The listing builds one solid part. Answer for the finished solid, in the listing's coordinates (mm). Give positions to 0.01 mm unless a question says otherwise; leave off trailing zeros. Order: outer loops, then holes, each group sorted by start corner. A loop starts at its lowest first (then second) coordinate and runs counter-clockwise, first axis right, second up. Notation, with made-up numbers: (27.5, -15.5) -> (55.5, -15.5) arc R17 ccw to (55.5, -3.5) -> close; hole circle Ø10 at (13.25, -13.5). An arc over 180 degrees is marked (long way). Write item = value, one per line. Start each with the question number.
Autodesk Inventor part; units mm, degrees
ref_plane "YZ Plane" through (0, 0, 0) normal (1, 0, 0) x (0, 1, 0)
ref_plane "XZ Plane" through (0, 0, 0) normal (0, 1, 0) x (-1, 0, 0)
ref_plane "XY Plane" through (0, 0, 0) normal (0, 0, 1) x (1, 0, 0)
sketch "スケッチ1" plane through (0, 0, 0) normal (1, 0, 0) x (0, 1, 0)
  circle A0 centre (0, 0) radius 15
  dimension "d0" = 30
extrude "押し出し1" add sketch "スケッチ1" along normal blind 10
sketch "スケッチ2" plane through (10, 0, 0) normal (1, 0, 0) x (0, 0, -1)
  circle A0 centre (0, 0) radius 16
  dimension "d3" = 32
extrude "押し出し2" add sketch "スケッチ2" along normal blind 1
sketch "スケッチ3" plane through (0, 0, 0) normal (-1, 0, 0) x (0, 0, 1)
  circle A0 centre (0, 0) radius 16
  dimension "d6" = 32
extrude "押し出し3" add sketch "スケッチ3" along normal blind 1
sketch "スケッチ4" plane through (-1, 0, 0) normal (-1, 0, 0) x (0, 0, 1)
  circle A0 centre (0, 0) radius 6
  dimension "d9" = 12
extrude "押し出し4" cut sketch "スケッチ4" against normal blind 12
properties part number "type2" material "アセタール樹脂、白"
Item 1: Consider L1, parallel to X at y = -14, z = -5.5; L2, parallel to Y at x = 1.25, z = 4; L3, parallel to Z at x = 8.25, y = -0.5. Determine where each line is inside the solid, lowest interval first. Write a range as from..to.
Item 2: A cutting plane is placed at D-D, the plane y = -12. Write down the section's boundary in (x, z).
Item 3: Flat-ended cylindrical pins translate along their axes: pin 1 (2 mm diameter, centred on x = 6, y = -7.5, fed in from -Z); pin 2 (3 mm diameter, centred on x = 3.5, y = 3, fed in from +Z); pin 3 (4 mm diameter, centred on x = 7, z = 2, fed in from +Y). Find the tip coordinate at first contact, or state that the pin passes through.
Item 4: A cutting plane is placed at A-A, the plane z = 0. Write down the section's boundary in (x, y).
Item 5: A cutting plane is placed at C-C, the plane x = 6. Write down the section's boundary in (y, z).
Item 6: The mould has two halves that part along Y. Classify faces 1 (the flat face through (-1, 0, 7)), 2 (the cylindrical face through (4.93, -14.985, -0.66)), 3 (the cylindrical face through (5, 0, -6)): +Y half, -Y half, draft (parallel to the pull), parting line (faces both ways), or undercut.
Check values:
q1.L1 = -1..0, 10..11
q1.L2 = -14.46..-4.47, 4.47..14.46
q1.L3 = -14.99..-5.98, 5.98..14.99
q2.outline = (-1, -10.58) -> (0, -10.58) -> (0, -9) -> (10, -9) -> (10, -10.58) -> (11, -10.58) -> (11, 10.58) -> (10, 10.58) -> (10, 9) -> (0, 9) -> (0, 10.58) -> (-1, 10.58) -> close
q3.pin_1 = -13.52
q3.pin_2 = 14.92
q3.pin_3 = 15
q4.outline = (-1, -16) -> (0, -16) -> (0, -15) -> (10, -15) -> (10, -16) -> (11, -16) -> (11, -6) -> (-1, -6) -> close; (-1, 6) -> (11, 6) -> (11, 16) -> (10, 16) -> (10, 15) -> (0, 15) -> (0, 16) -> (-1, 16) -> close
q5.outline = circle Ø30 at (0, 0); hole circle Ø12 at (0, 0)
q6.face_1 = draft
q6.face_2 = parting line
q6.face_3 = undercut
